Verification items for this drawing (mm, ordinates from the low corner). Coordinates: 2 decimals unless noted, no trailing zeros. Write each loop counter-clockwise with the first axis right and the second up, starting at its lowest first coordinate (ties: lowest second). Pieces come first, ordered by that corner, then holes. Notation, with made-up numbers: M 55,5 L 108,5 A21 cw 108,40 Z; hole C 41.5,-14.5 d7. An arc over 180 degrees is marked long. Write each question's results on one line, items separated by ' | '.
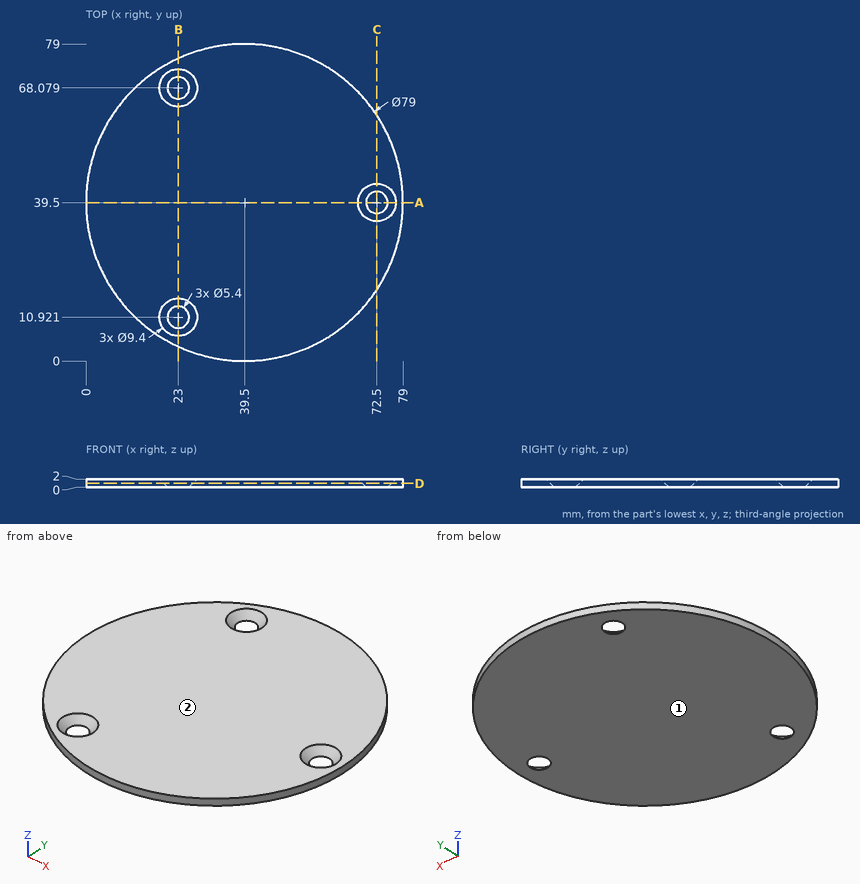
Q1. Mould release check, pull along Z, two halves, no side actions. Record for the marked faces 1 and 2: pulls with the +Z half, pulls with the -Z half, needs draft (parallel to the pull), parting line crosses it, or undercut.
Geometry check:
face 1: pulls with the -Z half | face 2: pulls with the +Z half
Q2. Depth check by flat-ended pin: P1, Ø1, axis at x = 10, z = 0.5, coming from the +Y side; P2, Ø1, axis at y = 47, z = 0.5, coming from the +X side (3 decimals); P3, Ø1, axis at y = 69.5, z = 0.5, coming from the +X side. Enter the tip coordinate at first touch or a pass-through.
Geometry check:
P1: stops at y = 66.32 | P2: stops at x = 78.375 | P3: stops at x = 65.77
Q3. Sectioned sample at A-A on y = 39.5. Record the cut outline in (x, z).
Geometry check:
outline: M 0,0 L 69.8,0 L 67.8,2 L 0,2 Z; M 75.2,0 L 79,0 L 79,2 L 77.2,2 Z
Q4. Scan lines: probe 1 along X at (y, z) = (65.5, 0.35) (1 decimal); probe 2 along X at (y, z) = (40.5, 1.6); probe 3 along Y at (x, z) = (24.5, 1.3). Record each from-to range of solid material in increasing order.
Geometry check:
probe 1: x = 9.8 to 21.4, 24.6 to 69.2 | probe 2: x = 0.01 to 68.32, 76.68 to 78.99 | probe 3: y = 2.96 to 7.21, 14.63 to 64.37, 71.79 to 76.04
Q5. Sectioned sample at B-B on x = 23. Record the cut outline in (y, z), and give its area (3 significant figures).
Geometry check:
outline: M 3.61,0 L 8.22,0 L 6.22,2 L 3.61,2 Z; M 13.62,0 L 65.38,0 L 63.38,2 L 15.62,2 Z; M 70.78,0 L 75.39,0 L 75.39,2 L 72.78,2 Z | area: 114 mm2
Q6. Sectioned sample at D-D on z = 0.9. Record the cut outline in (x, y), and give its area (3 significant figures).
Geometry check:
outline: C 39.5,39.5 d79; hole C 23,10.92 d7.2; hole C 23,68.08 d7.2; hole C 72.5,39.5 d7.2 | area: 4,780 mm2
Q7. Sectioned sample at C-C on x = 72.5. Record the cut outline in (y, z).
Geometry check:
outline: M 17.79,0 L 36.8,0 L 34.8,2 L 17.79,2 Z; M 42.2,0 L 61.21,0 L 61.21,2 L 44.2,2 Z
